```python
from build123d import *

# Parameters (mm, degrees)
F0_W     = 380
F0_H     = 10
F0_W_2   = 10
F0_H_2   = 120
F1_DEPTH = 300


with BuildPart() as f1:
    # F0 (on Top) → F1 (new body)
    with BuildSketch(Plane.XY):
        with Locations((190, -5)):
            Rectangle(F0_W, F0_H)
        Polygon((380, -10), (0, -10), (0, -150), (185, -182.620491), (185, -62.620491), (195, -62.620491), (195, -182.620491), (380, -150), align=None)
        with Locations((190, -122.620491)):
            Rectangle(F0_W_2, F0_H_2)
    extrude(amount=F1_DEPTH)


solid = f1.part
```
Part model, mm, in its own coordinate system. Round coordinates to 2 decimals unless told otherwise and drop trailing zeros. Write each loop counter-clockwise with the first axis right and the second up, starting at its lowest first coordinate (ties: lowest second). Pieces come first, ordered by that corner, then holes.
Item 1: Cut at C-C, the plane y = -170. Give the cut face in (x, z), plus the area to 3 significant figures.
Results:
outline: (113.43, 0) - (266.57, 0) - (266.57, 300) - (113.43, 300) - close
area: 45,900 mm2
Item 2: Drop a flat-ended pin along its axis: pin 1 Ø1.5 at (x, z) = (118, 67) entering from +Y. Give the stop position or say it passes through.
Results:
pin 1: stops at y = 0
Item 3: Probe L1, parallel to Y at x = 163, z = 257.5; L2, parallel to Y at x = 183.5, z = 138. List the from-to ranges inside material, lowest first.
Results:
L1: y = -178.74 to 0
L2: y = -182.36 to 0
Item 4: Cut at A-A, the plane z = 125.5. Give the cut face in (x, y).
Results:
outline: (0, -150) - (185, -182.62) - (195, -182.62) - (380, -150) - (380, 0) - (0, 0) - close
Item 5: Cut at B-B, the plane x = 52. Give the cut face in (y, z), plus the area to 3 significant figures.
Results:
outline: (-159.17, 0) - (0, 0) - (0, 300) - (-159.17, 300) - close
area: 47,800 mm2
